Autodesk Inventor part; units mm, degrees
ref_plane "YZ Plane" through (0, 0, 0) normal (1, 0, 0) x (0, 1, 0)
ref_plane "XZ Plane" through (0, 0, 0) normal (0, 1, 0) x (-1, 0, 0)
ref_plane "XY Plane" through (0, 0, 0) normal (0, 0, 1) x (1, 0, 0)
sketch "Sketch1" plane through (0, 0, 0) normal (0, 1, 0) x (-1, 0, 0)
  line L0 (0, -42) -> (0, 42)
  line L1 (-216, 0) -> (71, 0)
  circle A0 centre (0, 0) radius 16
  circle A1 centre (0, 0) radius 20
  arc A2 (0, -30) -> (0, 30) centre (0, 0) ccw
  line L2 (0, 30) -> (-60, 30)
  arc A3 (-75, 15) -> (-60, 30) centre (-75, 30) ccw
  line L3 (-75, 15) -> (-160, 15)
  arc A4 (-160, 15) -> (-160, -15) centre (-160, 0) ccw
  line L4 (0, -30) -> (-60, -30)
  arc A5 (-60, -30) -> (-75, -15) centre (-75, -30) ccw
  line L5 (-75, -15) -> (-160, -15)
  circle A6 centre (-160, 0) radius 5
  circle A7 centre (-80, 0) radius 5
  point P0 (0, 20)
  point P1 (0, 16)
  point P2 (-16, 0)
  point P3 (-20, 0)
  dimension "d0" = 30
  dimension "d1" = 40
  dimension "d2" = 4
  dimension "d3" = 10
  dimension "d4" = 80
  dimension "d5" = 60
  dimension "d6" = 160
  dimension "d8" = 15
  dimension "d10" = 15
extrude "Extrusion1" add sketch "Sketch1" along normal blind 6 contours L4 A5 L5 A4 L1 A6 A7 A1 L0 | L0 A1 L1 A2 | A1 L1 A0 L0 | L0 A0 L1 A1 | L1 A1 L0 A2 | A1 L0 A0 L1 | L1 A7 A6 A4 L3 A3 L2 L0 A1 | L1 A0 L0 A1
extrude "Extrusion2" add sketch "Sketch1" against normal blind 20 contours A1 L1 A0 L0 | L0 A0 L1 A1 | A1 L0 A0 L1 | L1 A0 L0 A1
extrude "Extrusion3" cut sketch "Sketch1" along normal through all contours A1 L1 A0 L0 | L0 A0 L1 A1 | L1 A0 L0 A1 | L1 A0 L0 picked at (-18.3658, -2.6703) picked at (17.7056, -5.5628) picked at (18.4995, 1.4835) picked at (-10.5329, 1.1868)
properties part number "Shared Sketch"
CAD build for the part. Positions are in the model's coordinates, mm. A direction names the side the tool comes from. Give positions to 0.01 mm unless a question says otherwise; leave off trailing zeros. Order: outer loops, then holes, each group sorted by start corner. A loop starts at its lowest first (then second) coordinate and runs counter-clockwise, first axis right, second up. Notation, with made-up numbers: (27, 0) - (36, 0) arc R23 ccw to (36, 37) - close; hole circle Ø9 at (41, 79.25). An arc over 180 degrees is marked (long way). Answer in a Markdown table with one row per item.
1. Saw through at C-C, the plane y = 3. Give the cut face in (x, z), plus the area to 3 significant figures.
Data:
| item | result |
|---|---|
| outline | (0, -30) - (60, -30) arc R15 cw to (75, -15) - (160, -15) arc R15 ccw to (160, 15) - (75, 15) arc R15 cw to (60, 30) - (0, 30) arc R30 ccw to start; hole (0, 16) - (0, 20) arc R20 ccw (long way) to (20, 0) - (16, 0) arc R16 ccw to start; hole circle Ø10 at (80, 0); hole circle Ø10 at (160, 0) |
| area | 7,160 mm² |
2. Tool access for faces 1 (the flat face through (117, 3, 15)), 2 (the flat face through (8.98, -20, 13.43)), 3 (the flat face through (117, 3, -15)), 4 (the cylindrical face through (4.336, -9.86, -19.524)), 5 (the flat face through (0, 3, 18)): list every direction of +Z, -Z, +X, -X, +Y, -Y with a clear straight run to the whole face (end or side of a thin tool).
Data:
| item | result |
|---|---|
| face 1 | +Z, +X, +Y, -Y |
| face 2 | +Z, -Z, +X, -X, -Y |
| face 3 | -Z, +X, +Y, -Y |
| face 4 | -Y |
| face 5 | +Y |
3. Pull direction Z, two halves, no side cores. Call faces 6 (the flat face through (30, 3, 30)), 7 (the cylindrical face through (175, 3, 0)), 8 (the cylindrical face through (3.47, -10.07, 15.62)): pulls with the +Z half, pulls with the -Z half, needs draft (parallel to the pull), parting line crosses it, or undercut.
Data:
| item | result |
|---|---|
| face 6 | pulls with the +Z half |
| face 7 | parting line crosses it |
| face 8 | undercut |
4. Probe probe 1 along Z at (x, y) = (80, 2.3); probe 2 along Z at (x, y) = (0, -9); probe 3 along X at (y, z) = (3, 3.5). List the from-to ranges inside material, lowest first. Write a range as [from, to].
Data:
| item | result |
|---|---|
| probe 1 | z = [-15, -5], [5, 15] |
| probe 2 | z = [-20, -16], [16, 20] |
| probe 3 | x = [-29.8, -19.69], [15.61, 76.43], [83.57, 156.43], [163.57, 174.59] |
5. Saw through at A-A, the plane x = 80. Give the cut face in (y, z), plus the area to 3 significant figures.
Data:
| item | result |
|---|---|
| outline | (0, -15) - (6, -15) - (6, -5) - (0, -5) - close; (0, 5) - (6, 5) - (6, 15) - (0, 15) - close |
| area | 120 mm² |
6. Flat gauge pins, fed straight in: pin 1 (2 mm diameter, centred on y = 3.5, z = 17.5, fed in from -X); pin 2 (1.5 mm diameter, centred on x = 146, z = -8.5, fed in from -Y); pin 3 (2 mm diameter, centred on y = -8.5, z = 1, fed in from -X). Where does each tip first touch, or does it go through?
Data:
| item | result |
|---|---|
| pin 1 | stops at x = -25.05 |
| pin 2 | stops at y = 0 |
| pin 3 | stops at x = -20 |
